Source: CAD feature listing. Evaluate the final solid. Frame: model axes, mm. Face numbers are marked on the shaded views. A direction names the side the tool comes from. Round coordinates to 2 decimals unless told otherwise and drop trailing zeros. Loops run counter-clockwise (first coordinate to the right, second up) from the corner with the lowest first, then second, coordinate; pieces in that order, holes last.
(1) Mould query, pull axis Y, two halves, no side actions, for the marked faces 1, 2, 3 and 4. Classes: pulls with the +Y half, pulls with the -Y half, needs draft (parallel to the pull), parting line crosses it, or undercut.
(2) Section A-A, the plane y = 29. Return the cut outline in (x, z), plus the area to 3 significant figures.
(3) Section C-C, the plane x = -29. Return the cut outline in (y, z), plus the area to 4 significant figures.
(4) Section B-B, the plane z = 9. Return the cut outline in (x, y), plus the area to 3 significant figures.
(5) First-contact query: pin 1 Ø1.5 at (x, z) = (-18.5, 7) entering from -Y; pin 2 Ø3 at (y, z) = (5.075, 16.595) entering from +X; pin 3 Ø10 at (x, y) = (-23, 22.5) entering from +Z; pin 4 Ø0.8 at (y, z) = (5.5, 16.5) entering from +X. Flat tips, straight axial feed; report the tip coordinate or a pass-through.
(6) Material intervals for probe 1 along Y at (x, z) = (-22, 0); probe 2 along Z at (x, y) = (-13.5, 49); probe 3 along Y at (x, z) = (-7.5, 12.75), sorted ascending.
(7) Set-up query: the marked faces 5, 6, 7 and 8. Return all of +Z, -Z, +X, -X, +Y, -Y with unobstructed straight access to the full face (end or side cutting, diameter ignored); none if empty.
(8) Section D-D, the plane y = 46. Return the cut outline in (x, z), plus the area to 3 significant figures.
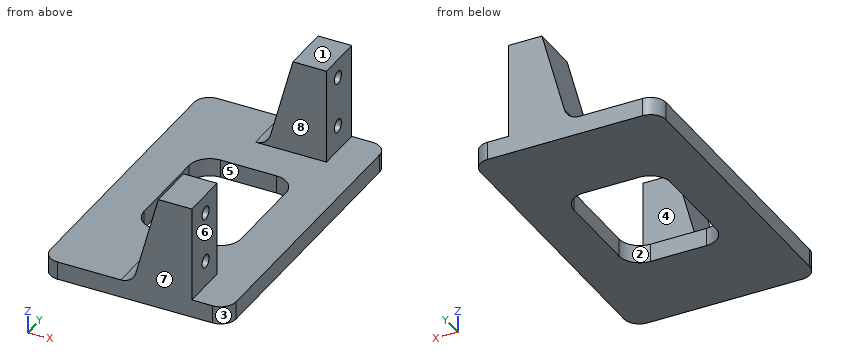
Autodesk Inventor part; units mm, degrees
ref_plane "YZ Plane" through (0, 0, 0) normal (1, 0, 0) x (0, 1, 0)
ref_plane "XZ Plane" through (0, 0, 0) normal (0, 1, 0) x (-1, 0, 0)
ref_plane "XY Plane" through (0, 0, 0) normal (0, 0, 1) x (1, 0, 0)
sketch "Base" plane through (0, 0, 0) normal (0, 0, 1) x (1, 0, 0)
  line L0 (0, 0) -> (-36, 0)
  line L1 (-36, 0) -> (-36, 59)
  line L2 (-36, 59) -> (0, 59)
  line L3 (0, 59) -> (0, 0)
  dimension "d0" = 36
  dimension "d1" = 59
extrude "Extrusion1" add sketch "Base" along normal mid plane 3.5
sketch "Attachment Towers" plane through (0, 0, 1.75) normal (0, 0, 1) x (1, 0, 0)
  line L0 (0, 29.5) -> (-7, 29.5) construction
  line L1 (-7, 29.5) -> (-7, 49.7) construction
  line L2 (-7, 29.5) -> (-7, 9.3) construction
  line L3 (-7, 49.7) -> (-13.5, 49.7)
  line L4 (-13.5, 49.7) -> (-13.5, 59)
  line L5 (-13.5, 59) -> (-7, 59)
  line L6 (-7, 59) -> (-7, 49.7)
  line L7 (-7, 9.3) -> (-13.5, 9.3)
  line L8 (-13.5, 9.3) -> (-13.5, 0)
  line L9 (-13.5, 0) -> (-7, 0)
  line L10 (-7, 0) -> (-7, 9.3)
  dimension "d41" = 7
  dimension "d44" = 40.4
  dimension "d45" = 6.5
  dimension "d46" = 9.3
extrude "Extrusion3" add sketch "Attachment Towers" along normal blind 18.5
sketch "Screw Holes" plane through (-7, 0, 1.75) normal (1, 0, 0) x (0, 0, -1)
  line L0 (0, 49.7) -> (0, 51.8) construction
  line L1 (0, 51.8) -> (-7.15, 51.8) construction
  circle A0 centre (-5.025, 53.925) radius 2.125 construction
  line L2 (-7.15, 51.8) -> (-7.15, 61.0367) construction
  line L3 (-2.9, 53.925) -> (-16.97, 53.925) construction
  circle A1 centre (-14.845, 53.925) radius 2.125 construction
  line L4 (-16.97, 51.8) -> (-16.97, 61.0367) construction
  circle A2 centre (-14.845, 53.925) radius 1.275
  circle A3 centre (-5.025, 53.925) radius 1.275
  line L5 (0, 29.5) -> (-35.6681, 29.5) construction
  circle A4 centre (-14.845, 5.075) radius 1.275
  circle A5 centre (-5.025, 5.075) radius 1.275
  dimension "d18" = 4.25
  dimension "d15" = 2.1
  dimension "d16" = 7.15
  dimension "d20" = 14.07
  dimension "d21" = 4.25
  dimension "d22" = 2.55
  dimension "d23" = 2.55
extrude "Extrusion4" cut sketch "Screw Holes" against normal blind 4
draft "FaceDraft1" angle 15 pull direction (0, 0, 1) faces at (-13.5, 6.2, 7.9167) (-13.5, 55.9, 7.9167) fixed edges at (-13.5, 4.65, 20.25) (-13.5, 54.35, 20.25)
sketch "Sketch5" plane through (0, 0, 1.75) normal (0, 0, 1) x (1, 0, 0)
  line L0 (-36, 29.5) -> (0, 29.5) construction
  line L1 (-23.4056, 41.836) -> (-12.5944, 41.836)
  line L2 (-8.5944, 37.836) -> (-8.5944, 21.164)
  line L3 (-12.5944, 17.164) -> (-23.4056, 17.164)
  line L4 (-27.4056, 21.164) -> (-27.4056, 37.836)
  line L5 (-27.4056, 41.836) -> (-8.5944, 17.164) construction
  line L6 (-8.5944, 41.836) -> (-27.4056, 17.164) construction
  arc A0 (-27.4056, 21.164) -> (-23.4056, 17.164) centre (-23.4056, 21.164) ccw
  arc A1 (-12.5944, 17.164) -> (-8.5944, 21.164) centre (-12.5944, 21.164) ccw
  arc A2 (-8.5944, 37.836) -> (-12.5944, 41.836) centre (-12.5944, 37.836) ccw
  arc A3 (-23.4056, 41.836) -> (-27.4056, 37.836) centre (-23.4056, 37.836) ccw
  point P0 (-18, 29.5)
  dimension "d47" = 4
extrude "Extrusion5" cut sketch "Sketch5" against normal through all
fillet "Fillet1" radius 3 6 edges at (0, 0, 0) (0, 59, 0) (-36, 59, 0) (-36, 0, 0) (-18.4571, 4.65, 1.75) (-18.4571, 54.35, 1.75)
sketch "Axle Reference" plane through (-7, 0, 1.75) normal (1, 0, 0) x (0, 0, -1)
  circle A0 centre (-14.845, 5.075) radius 1.275 construction
  circle A1 centre (-5.025, 5.075) radius 1.275 construction
  line L0 (-9.935, 5.075) -> (-9.935, 39.375) construction
  line L1 (-9.935, 53.925) -> (-9.935, 39.375) construction
  line L2 (-9.935, 39.375) -> (0, 39.375) construction
  line L3 (0, 56) -> (0, 3) construction
  circle A2 centre (-14.845, 5.075) radius 1.275 construction
  line L4 (-14.845, 5.075) -> (-5.025, 5.075) construction
  point P0 (1.75, 0)
  dimension "d48" = 34.3
  dimension "d49" = 14.55
  dimension "d50" = 9.935
  dimension "d51" = 9.82
properties part number "MG996R Attachment Test"
Output values:
1. face 1: needs draft
1. face 2: undercut
1. face 3: pulls with the -Y half
1. face 4: undercut
2. outline: (-36, -1.75) - (-27.41, -1.75) - (-27.41, 1.75) - (-36, 1.75) - close; (-8.59, -1.75) - (0, -1.75) - (0, 1.75) - (-8.59, 1.75) - close
2. area: 60.2 mm2
3. outline: (0, -1.75) - (59, -1.75) - (59, 1.75) - (0, 1.75) - close
3. area: 206.5 mm2
4. outline: (-16.51, 0) - (-7, 0) - (-7, 9.3) - (-16.51, 9.3) - close; (-16.51, 49.7) - (-7, 49.7) - (-7, 59) - (-16.51, 59) - close
4. area: 177 mm2
5. pin 1: passes through
5. pin 2: stops at x = -7
5. pin 3: stops at z = 1.75
5. pin 4: stops at x = -11
6. probe 1: y = 0 to 17.16, 41.84 to 59
6. probe 2: z = -1.75 to 1.75
6. probe 3: y = 0 to 9.3, 49.7 to 59
7. face 5: +Z, -Z
7. face 6: +Z, +X, +Y, -Y
7. face 7: +Z, -Z, +X, -X, -Y
7. face 8: +Z, +X, -X
8. outline: (-36, -1.75) - (0, -1.75) - (0, 1.75) - (-36, 1.75) - close
8. area: 126 mm2
